Verification items for the finished model (mm, model axes). Face numbers are marked on the shaded views. Round coordinates to 2 decimals unless told otherwise and drop trailing zeros. Loops run counter-clockwise (first coordinate to the right, second up) from the corner with the lowest first, then second, coordinate; pieces in that order, holes last. Notation, with made-up numbers: (-1, 22) -> (17, 22) arc R29 cw to (17, 54) -> close; hole circle Ø11 at (1, 16). An arc over 180 degrees is marked (long way). Write item = value, one per line.
```python
from build123d import *

# Parameters (mm, degrees)
SKETCH1_R           = 2
BOSS_EXTRUDE1_DEPTH = 5
CHAMFER1_SIZE       = 0.15


with BuildPart() as part:
    # Sketch1 → Boss-Extrude1 (new, symmetric)
    with BuildSketch(Plane.XY):
        with BuildLine():
            Line((0, 4), (-4, 4))
            Line((-4, 4), (-4, -4))
            Line((-4, -4), (0, -4))
            ThreePointArc((0, -4), (4, 0), (0, 4))
        make_face()
        Circle(SKETCH1_R, mode=Mode.SUBTRACT)
    extrude(amount=BOSS_EXTRUDE1_DEPTH, both=True)

    # Chamfer1
    chamfer1_edges = [part.edges().sort_by_distance(p)[0] for p in [
        (-2, 0, -5),
        (-2, 0, 5),
        (-4, 0, 5),
        (-2, -4, 5),
        (4, 0, 5),
        (-2, -4, -5),
        (-4, 0, -5),
        (-2, 4, -5),
        (4, 0, -5),
        (-4, -4, 0),
        (-4, 4, 0),
        (-2, 4, 5),
    ]]
    chamfer(chamfer1_edges, length=CHAMFER1_SIZE)


solid = part.part
```
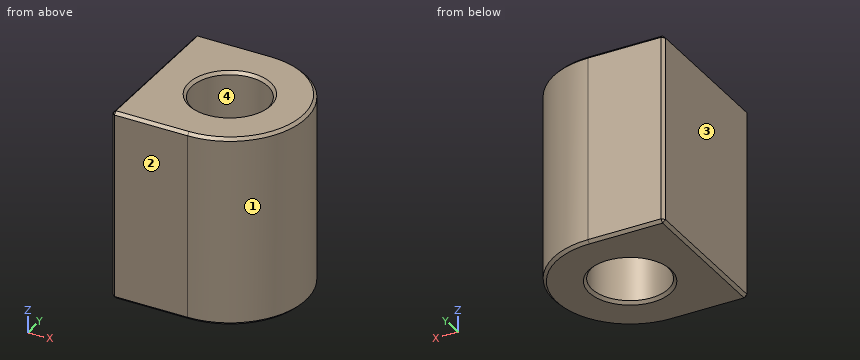
(1) Sectioned sample at B-B, the plane y = 0. Record the cut outline in (x, z), and give its area (3 significant figures).
Filled sheet:
outline = (-4, -4.85) -> (-3.85, -5) -> (-2.15, -5) -> (-2, -4.85) -> (-2, 4.85) -> (-2.15, 5) -> (-3.85, 5) -> (-4, 4.85) -> close; (2, -4.85) -> (2.15, -5) -> (3.85, -5) -> (4, -4.85) -> (4, 4.85) -> (3.85, 5) -> (2.15, 5) -> (2, 4.85) -> close
area = 39.9 mm2
(2) Sectioned sample at A-A, the plane z = 2.25. Record the cut outline in (x, y).
Filled sheet:
outline = (-4, -3.85) -> (-3.85, -4) -> (0, -4) arc R4 ccw to (0, 4) -> (-3.85, 4) -> (-4, 3.85) -> close; hole circle Ø4 at (0, 0)
(3) Go/stop test with a flat-tipped pin: pin 1 Ø1 at (y, z) = (-1.5, 4) entering from +X. Record where the tip stops, or that it passes through.
Filled sheet:
pin_1 = 3.87
(4) Draft check along Y on the marked faces 1, 2, 3 and 4. Enter one of: released by +Y, released by -Y, zero draft, split by the parting line, or undercut.
Filled sheet:
face_1 = split by the parting line
face_2 = released by -Y
face_3 = zero draft
face_4 = undercut
(5) Material ranges on probe 1 along Y at (x, z) = (-1.75, -0.25); probe 2 along Y at (x, z) = (0.5, 2.25); probe 3 along X at (y, z) = (-1.25, -1.25), recorded low to high. Write a range as from..to.
Filled sheet:
probe_1 = -4..-0.97, 0.97..4
probe_2 = -3.97..-1.94, 1.94..3.97
probe_3 = -4..-1.56, 1.56..3.8
